Geometry: final body of the model. Coordinates: model frame, mm. Give positions to 0.01 mm unless a question says otherwise; leave off trailing zeros. Return JSON: item names as keys, results as strings.
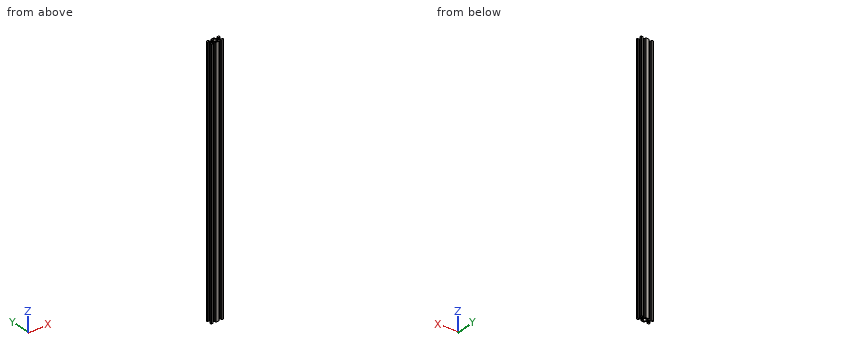
from build123d import *

# Parameters (mm, degrees)
SKETCH_1_R      = 2.5
EXTRUDE_1_DEPTH = 800


with BuildPart() as part:
    # Эскиз1 → Бобышка-Вытянуть1 (new body)
    with BuildSketch(Plane.XY):
        with BuildLine():
            Line((-18.5, 14.076873633), (-14.75, 14.076873633))
            Line((-14.75, 14.076873633), (-13.1, 12.076873633))
            Line((-13.1, 12.076873633), (-14.65, 12.076873633))
            ThreePointArc((-14.65, 12.076873633), (-14.720710678, 12.047584311), (-14.75, 11.976873633))
            Line((-14.75, 11.976873633), (-14.75, 10.726998833))
            ThreePointArc((-14.75, 10.726998833), (-14.728880127, 10.583214884), (-14.667304703, 10.451577729))
            Line((-14.667304703, 10.451577729), (-13.248222071, 8.301452529))
            ThreePointArc((-13.248222071, 8.301452529), (-13.067866147, 8.136583642), (-12.830917368, 8.076873633))
            Line((-12.830917368, 8.076873633), (-7.169082632, 8.076873633))
            ThreePointArc((-7.169082632, 8.076873633), (-6.932133853, 8.136583642), (-6.751777929, 8.301452529))
            Line((-6.751777929, 8.301452529), (-5.332695297, 10.451577729))
            ThreePointArc((-5.332695297, 10.451577729), (-5.271119873, 10.583214884), (-5.25, 10.726998833))
            Line((-5.25, 10.726998833), (-5.25, 11.976873633))
            ThreePointArc((-5.25, 11.976873633), (-5.279289322, 12.047584311), (-5.35, 12.076873633))
            Line((-5.35, 12.076873633), (-6.9, 12.076873633))
            Line((-6.9, 12.076873633), (-5.25, 14.076873633))
            Line((-5.25, 14.076873633), (5.25, 14.076873633))
            Line((5.25, 14.076873633), (6.9, 12.076873633))
            Line((6.9, 12.076873633), (5.35, 12.076873633))
            ThreePointArc((5.35, 12.076873633), (5.279289322, 12.047584311), (5.25, 11.976873633))
            Line((5.25, 11.976873633), (5.25, 10.726998833))
            ThreePointArc((5.25, 10.726998833), (5.271119873, 10.583214884), (5.332695297, 10.451577729))
            Line((5.332695297, 10.451577729), (6.751777929, 8.301452529))
            ThreePointArc((6.751777929, 8.301452529), (6.932133853, 8.136583642), (7.169082632, 8.076873633))
            Line((7.169082632, 8.076873633), (12.830917368, 8.076873633))
            ThreePointArc((12.830917368, 8.076873633), (13.067866147, 8.136583642), (13.248222071, 8.301452529))
            Line((13.248222071, 8.301452529), (14.667304703, 10.451577729))
            ThreePointArc((14.667304703, 10.451577729), (14.728880127, 10.583214884), (14.75, 10.726998833))
            Line((14.75, 10.726998833), (14.75, 11.976873633))
            ThreePointArc((14.75, 11.976873633), (14.720710678, 12.047584311), (14.65, 12.076873633))
            Line((14.65, 12.076873633), (13.1, 12.076873633))
            Line((13.1, 12.076873633), (14.75, 14.076873633))
            Line((14.75, 14.076873633), (18.5, 14.076873633))
            ThreePointArc((18.5, 14.076873633), (19.560660172, 13.637533805), (20, 12.576873633))
            Line((20, 12.576873633), (20, 8.826873633))
            Line((20, 8.826873633), (18, 7.176873633))
            Line((18, 7.176873633), (18, 8.726873633))
            ThreePointArc((18, 8.726873633), (17.970710678, 8.797584311), (17.9, 8.826873633))
            Line((17.9, 8.826873633), (16.6501252, 8.826873633))
            ThreePointArc((16.6501252, 8.826873633), (16.50634125, 8.80575376), (16.374704096, 8.744178337))
            Line((16.374704096, 8.744178337), (14.224578896, 7.325095704))
            ThreePointArc((14.224578896, 7.325095704), (14.059710009, 7.14473978), (14, 6.907791001))
            Line((14, 6.907791001), (14, 1.245956265))
            ThreePointArc((14, 1.245956265), (14.059710009, 1.009007486), (14.224578896, 0.828651562))
            Line((14.224578896, 0.828651562), (16.374704096, -0.59043107))
            ThreePointArc((16.374704096, -0.59043107), (16.50634125, -0.652006494), (16.6501252, -0.673126367))
            Line((16.6501252, -0.673126367), (17.9, -0.673126367))
            ThreePointArc((17.9, -0.673126367), (17.970710678, -0.643837045), (18, -0.573126367))
            Line((18, -0.573126367), (18, 0.976873633))
            Line((18, 0.976873633), (20, -0.673126367))
            Line((20, -0.673126367), (20, -4.423126367))
            ThreePointArc((20, -4.423126367), (19.560660172, -5.483786539), (18.5, -5.923126367))
            Line((18.5, -5.923126367), (14.75, -5.923126367))
            Line((14.75, -5.923126367), (13.1, -3.923126367))
            Line((13.1, -3.923126367), (14.65, -3.923126367))
            ThreePointArc((14.65, -3.923126367), (14.720710678, -3.893837045), (14.75, -3.823126367))
            Line((14.75, -3.823126367), (14.75, -2.573251567))
            ThreePointArc((14.75, -2.573251567), (14.728880127, -2.429467617), (14.667304703, -2.297830463))
            Line((14.667304703, -2.297830463), (13.248222071, -0.147705263))
            ThreePointArc((13.248222071, -0.147705263), (13.067866147, 0.017163624), (12.830917368, 0.076873633))
            Line((12.830917368, 0.076873633), (7.169082632, 0.076873633))
            ThreePointArc((7.169082632, 0.076873633), (6.932133853, 0.017163624), (6.751777929, -0.147705263))
            Line((6.751777929, -0.147705263), (5.332695297, -2.297830463))
            ThreePointArc((5.332695297, -2.297830463), (5.271119873, -2.429467617), (5.25, -2.573251567))
            Line((5.25, -2.573251567), (5.25, -3.823126367))
            ThreePointArc((5.25, -3.823126367), (5.279289322, -3.893837045), (5.35, -3.923126367))
            Line((5.35, -3.923126367), (6.9, -3.923126367))
            Line((6.9, -3.923126367), (5.25, -5.923126367))
            Line((5.25, -5.923126367), (-5.25, -5.923126367))
            Line((-5.25, -5.923126367), (-6.9, -3.923126367))
            Line((-6.9, -3.923126367), (-5.35, -3.923126367))
            ThreePointArc((-5.35, -3.923126367), (-5.279289322, -3.893837045), (-5.25, -3.823126367))
            Line((-5.25, -3.823126367), (-5.25, -2.573251567))
            ThreePointArc((-5.25, -2.573251567), (-5.271119873, -2.429467617), (-5.332695297, -2.297830463))
            Line((-5.332695297, -2.297830463), (-6.751777929, -0.147705263))
            ThreePointArc((-6.751777929, -0.147705263), (-6.932133853, 0.017163624), (-7.169082632, 0.076873633))
            Line((-7.169082632, 0.076873633), (-12.830917368, 0.076873633))
            ThreePointArc((-12.830917368, 0.076873633), (-13.067866147, 0.017163624), (-13.248222071, -0.147705263))
            Line((-13.248222071, -0.147705263), (-14.667304703, -2.297830463))
            ThreePointArc((-14.667304703, -2.297830463), (-14.728880127, -2.429467617), (-14.75, -2.573251567))
            Line((-14.75, -2.573251567), (-14.75, -3.823126367))
            ThreePointArc((-14.75, -3.823126367), (-14.720710678, -3.893837045), (-14.65, -3.923126367))
            Line((-14.65, -3.923126367), (-13.1, -3.923126367))
            Line((-13.1, -3.923126367), (-14.75, -5.923126367))
            Line((-14.75, -5.923126367), (-18.5, -5.923126367))
            ThreePointArc((-18.5, -5.923126367), (-19.560660172, -5.483786539), (-20, -4.423126367))
            Line((-20, -4.423126367), (-20, -0.673126367))
            Line((-20, -0.673126367), (-18, 0.976873633))
            Line((-18, 0.976873633), (-18, -0.573126367))
            ThreePointArc((-18, -0.573126367), (-17.970710678, -0.643837045), (-17.9, -0.673126367))
            Line((-17.9, -0.673126367), (-16.6501252, -0.673126367))
            ThreePointArc((-16.6501252, -0.673126367), (-16.50634125, -0.652006494), (-16.374704096, -0.59043107))
            Line((-16.374704096, -0.59043107), (-14.224578896, 0.828651562))
            ThreePointArc((-14.224578896, 0.828651562), (-14.059710009, 1.009007486), (-14, 1.245956265))
            Line((-14, 1.245956265), (-14, 6.907791001))
            ThreePointArc((-14, 6.907791001), (-14.059710009, 7.14473978), (-14.224578896, 7.325095704))
            Line((-14.224578896, 7.325095704), (-16.374704096, 8.744178337))
            ThreePointArc((-16.374704096, 8.744178337), (-16.50634125, 8.80575376), (-16.6501252, 8.826873633))
            Line((-16.6501252, 8.826873633), (-17.9, 8.826873633))
            ThreePointArc((-17.9, 8.826873633), (-17.970710678, 8.797584311), (-18, 8.726873633))
            Line((-18, 8.726873633), (-18, 7.176873633))
            Line((-18, 7.176873633), (-20, 8.826873633))
            Line((-20, 8.826873633), (-20, 12.576873633))
            ThreePointArc((-20, 12.576873633), (-19.560660172, 13.637533805), (-18.5, 14.076873633))
        make_face()
        with Locations((-10, 4.076873633)):
            Circle(SKETCH_1_R, mode=Mode.SUBTRACT)
        with Locations((10, 4.076873633)):
            Circle(SKETCH_1_R, mode=Mode.SUBTRACT)
        with BuildLine():
            Line((-6, 6.220171901), (-6, 1.933575365))
            ThreePointArc((-6, 1.933575365), (-5.863556224, 1.30850383), (-5.479047434, 0.797148455))
            Line((-5.479047434, 0.797148455), (-0.652698289, -3.360817802))
            ThreePointArc((-0.652698289, -3.360817802), (0, -3.603199861), (0.652698289, -3.360817802))
            Line((0.652698289, -3.360817802), (5.479047434, 0.797148455))
            ThreePointArc((5.479047434, 0.797148455), (5.863556224, 1.30850383), (6, 1.933575365))
            Line((6, 1.933575365), (6, 6.220171901))
            ThreePointArc((6, 6.220171901), (5.863556224, 6.845243437), (5.479047434, 7.356598811))
            Line((5.479047434, 7.356598811), (0.652698289, 11.514565068))
            ThreePointArc((0.652698289, 11.514565068), (0, 11.756947128), (-0.652698289, 11.514565068))
            Line((-0.652698289, 11.514565068), (-5.479047434, 7.356598811))
            ThreePointArc((-5.479047434, 7.356598811), (-5.863556224, 6.845243437), (-6, 6.220171901))
        make_face(mode=Mode.SUBTRACT)
    extrude(amount=-EXTRUDE_1_DEPTH)


solid = part.part
Q1. Section query A-A, the plane z = -341.5. Count the separate pieces of the cut face and the enclosed holes in it, plus the area to 3 significant figures.
Answer key:
{"separate pieces": "1", "enclosed holes": "3", "area": "332 mm^2"}
Q2. Pin query (flat end, axial travel): P1, Ø0.5, axis at x = -14, z = -237.5, coming from the -Y side; P2, Ø1.2, axis at y = 0, z = -371.5, coming from the -X side; P3, Ø1.3, axis at y = 3, z = -376.5, coming from the -X side. Return the tip coordinate at first contact, or that it passes through.
Answer key:
{"P1": "stops at y = -5.32", "P2": "stops at x = -19.91", "P3": "stops at x = -14"}
Q3. Material intervals for probe 1 along X at (y, z) = (0.5, -742); probe 2 along X at (y, z) = (-4, -414); probe 3 along X at (y, z) = (4, -739.5), sorted ascending. Write a range as [from, to].
Answer key:
{"probe 1": "x = [-18.58, -18], [-14.72, -5.13], [5.13, 14.72], [18, 18.58]", "probe 2": "x = [-20, -13.16], [-6.84, 6.84], [13.16, 20]", "probe 3": "x = [-14, -12.5], [-7.5, -6], [6, 7.5], [12.5, 14]"}
